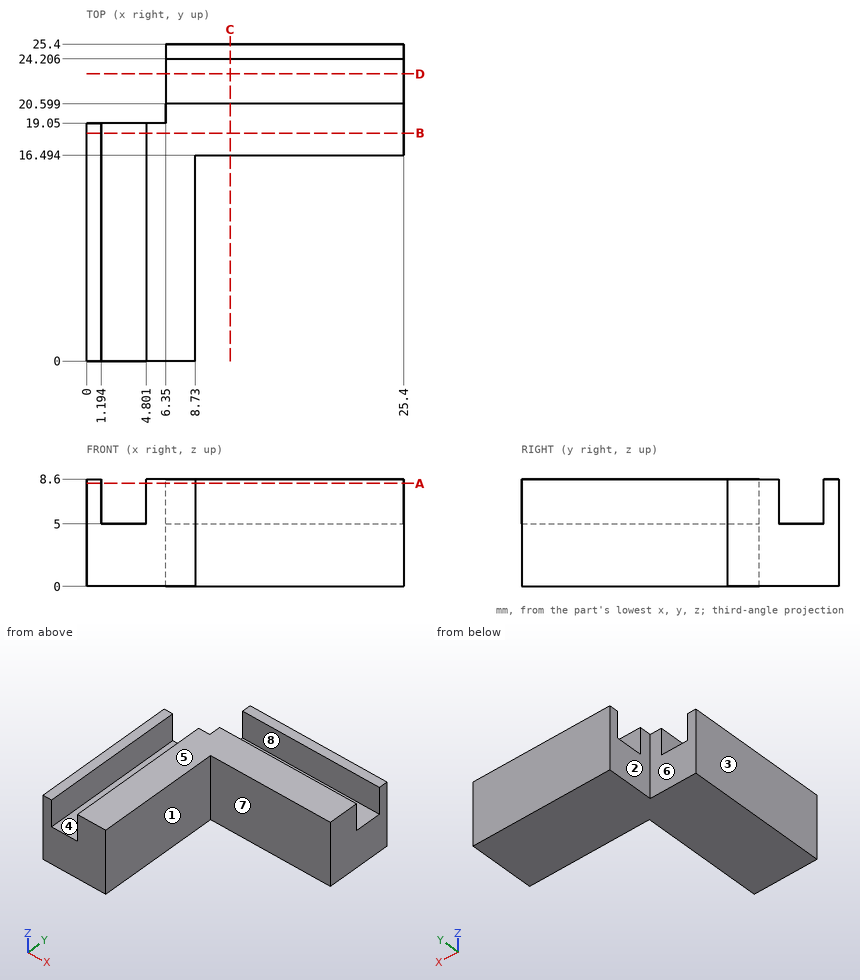
Design review of the part shown in the three views and the two pictorial views. Dimensions are in mm from the part's minimum x, y and z. A direction names the side the tool comes from. Round coordinates to 2 decimals unless told otherwise and drop trailing zeros. Write each loop counter-clockwise with the first axis right and the second up, starting at its lowest first coordinate (ties: lowest second). Pieces come first, ordered by that corner, then holes.
Item 1: We need section D-D on y = 23. Write out the cut boundary in (x, z).
Item 2: For probe 1 along Y at (x, z) = (18.5, 5.5); probe 2 along Y at (x, z) = (7, 5.5); probe 3 along X at (y, z) = (19, 7.75), list the stretches that pass through material, from the lowest coordinate up.
Item 3: For the marked faces 1, 2, 3 and 4, list the 3-axis set-ups (+Z, -Z, +X, -X, +Y, -Y) from which the entire face can be reached by the end or side of a thin tool; tool diameter is ignored.
Item 4: Clearance check with flat-ended pins moving along their axes: pin 1 Ø3 at (y, z) = (23, 2.5) entering from -X; pin 2 Ø4 at (x, z) = (15.5, 6) entering from -Y; pin 3 Ø4 at (y, z) = (9, 6.5) entering from +X. State where each tip first meets the part, or that it passes through.
Item 5: We need section A-A on z = 8.25. Write out the cut boundary in (x, y).
Item 6: We need section C-C on x = 11.5. Write out the cut boundary in (y, z).
Item 7: We need section B-B on y = 18.25. Write out the cut boundary in (x, z).
Item 8: The part is to be moulded in two halves that separate along Y. For the marked faces 5, 6, 7 and 8, say which applies: +Y half, -Y half, draft (parallel to the pull), parting line (faces both ways), or undercut.
Returned:
1. outline: (6.35, 0) - (25.4, 0) - (25.4, 5) - (6.35, 5) - close
2. probe 1: y = 16.49 to 20.6, 24.21 to 25.4
2. probe 2: y = 0 to 20.6, 24.21 to 25.4
2. probe 3: x = 0 to 1.19, 4.8 to 25.4
3. face 1: +Z, -Z, +X, -Y
3. face 2: +Z, -Z, -X, +Y
3. face 3: +Z, -Z, -X, +Y, -Y
3. face 4: +Z, +Y, -Y
4. pin 1: stops at x = 6.35
4. pin 2: stops at y = 16.49
4. pin 3: stops at x = 8.73
5. outline: (0, 0) - (1.19, 0) - (1.19, 19.05) - (0, 19.05) - close; (4.8, 0) - (8.73, 0) - (8.73, 16.49) - (25.4, 16.49) - (25.4, 20.6) - (6.35, 20.6) - (6.35, 19.05) - (4.8, 19.05) - close; (6.35, 24.21) - (25.4, 24.21) - (25.4, 25.4) - (6.35, 25.4) - close
6. outline: (16.49, 0) - (25.4, 0) - (25.4, 8.6) - (24.21, 8.6) - (24.21, 5) - (20.6, 5) - (20.6, 8.6) - (16.49, 8.6) - close
7. outline: (0, 0) - (25.4, 0) - (25.4, 8.6) - (4.8, 8.6) - (4.8, 5) - (1.19, 5) - (1.19, 8.6) - (0, 8.6) - close
8. face 5: draft
8. face 6: +Y half
8. face 7: -Y half
8. face 8: undercut
